Geometry: final body of the model. Coordinates: model frame, mm. Face numbers are marked on the shaded views. A direction names the side the tool comes from. Round coordinates to 2 decimals unless told otherwise and drop trailing zeros. Loops run counter-clockwise (first coordinate to the right, second up) from the corner with the lowest first, then second, coordinate; pieces in that order, holes last. Notation, with made-up numbers: (88.25, 30.5) -> (143.25, 30.5) arc R19 cw to (143.25, 55.5) -> close; hole circle Ø10 at (59, 17.25). An arc over 180 degrees is marked (long way). Answer in a Markdown table with one row per item.
Autodesk Inventor part; units mm, degrees
ref_plane "YZ Plane" through (0, 0, 0) normal (1, 0, 0) x (0, 1, 0)
ref_plane "XZ Plane" through (0, 0, 0) normal (0, 1, 0) x (-1, 0, 0)
ref_plane "XY Plane" through (0, 0, 0) normal (0, 0, 1) x (1, 0, 0)
sketch "Sketch11" plane through (0, 0, 0) normal (0, 1, 0) x (-1, 0, 0)
  circle A0 centre (0, 0) radius 26
  circle A1 centre (0, 0) radius 24
  circle A2 centre (0, 0) radius 31
  circle A3 centre (0, 0) radius 55
  line L0 (35.5726, 38.3198) -> (39.3254, 31.8198)
  line L1 (39.3254, 31.8198) -> (35.5726, 25.3198)
  line L2 (35.5726, 25.3198) -> (28.067, 25.3198)
  line L3 (28.067, 25.3198) -> (24.3143, 31.8198)
  line L4 (24.3143, 31.8198) -> (28.067, 38.3198)
  line L5 (28.067, 38.3198) -> (35.5726, 38.3198)
  line L6 (0, 0) -> (31.8198, 31.8198) construction
  line L7 (0, 0) -> (45, 0) construction
  line L8 (35.5726, 38.3198) -> (28.067, 25.3198) construction
  line L9 (28.067, 38.3198) -> (35.5726, 25.3198) construction
  line L10 (39.3254, 31.8198) -> (24.3143, 31.8198) construction
  line L11 (0, 52.6213) -> (0, 85)
  line L12 (0, 85) -> (-16, 85)
  line L13 (-16, 85) -> (-16, 52.6213)
  line L14 (0, 74.5) -> (120, 74.5)
  line L15 (120, 74.5) -> (120, 80)
  line L16 (120, 80) -> (0, 80)
  line L17 (0, 80) -> (0, 74.5)
  line L18 (120, 90.5) -> (120, 58.5)
  arc A4 (120, 58.5) -> (120, 90.5) centre (120, 74.5) ccw
  line L19 (-16, 52.6213) -> (0, 52.6213)
  line L20 (0, 52.6213) -> (-16, 52.6213)
  line L21 (-16, 52.6213) -> (-16, 44.6213)
  line L22 (-16, 44.6213) -> (0, 44.6213)
  line L23 (0, 44.6213) -> (0, 52.6213)
  dimension "oOuterDia" = 110
  dimension "oPipeDia" = 52
  dimension "oPipeWall" = 2
  dimension "oPipeLenght" = 5
  dimension "oKdia" = 45
  dimension "d70" = 45
  dimension "oSW" = 13
  dimension "oCenterTop" = 85
  dimension "d78" = 16
  dimension "oHandleLenght" = 120
  dimension "d80" = 5.5
  dimension "d81" = 32
  dimension "d82" = 5
  dimension "d86" = 8
extrude "Extrusion12" add sketch "Sketch11" along normal mid plane 52 contours A0
extrude "Extrusion13" add sketch "Sketch11" along normal mid plane 42 contours A2
extrude "Extrusion14" add sketch "Sketch11" along normal mid plane 22 contours L21 L22 L23 L11 A3 | A3 L11 L19 | L19 L23 L22 L21 | L0 L1 L2 L3 L4 L5
extrude "Extrusion15" add sketch "Sketch11" along normal mid plane 38 contours L0 L1 L2 L3 L4 L5
pattern_circular "Circular Pattern2" count 4 over 360 about axis through (0, 0, 0) along (0, 1, 0) of "Extrusion15"
revolve "Revolution1" add sketch "Sketch11" angle 360 about axis through (0, 0, 52.6213) along (0, 0, 1) contours L13 L12 L11 A3 | A3 L11 L19 | L19 L23 L22 L21
revolve "Revolution2" add sketch "Sketch11" angle 360 about axis through (0, 0, 74.5) along (-1, 0, 0) contours L11 L16 L15 L14
revolve "Revolution3" add sketch "Sketch11" angle 360 about axis through (-120, 0, 90.5) along (0, 0, -1) contours L15 L18 A4
equation "\"d65\" = -2 * oPipeLenght + oValveLenght"
properties part number "MANUAL SANITARY BUTTERFLY VALVE 304L DN50" material "304L"
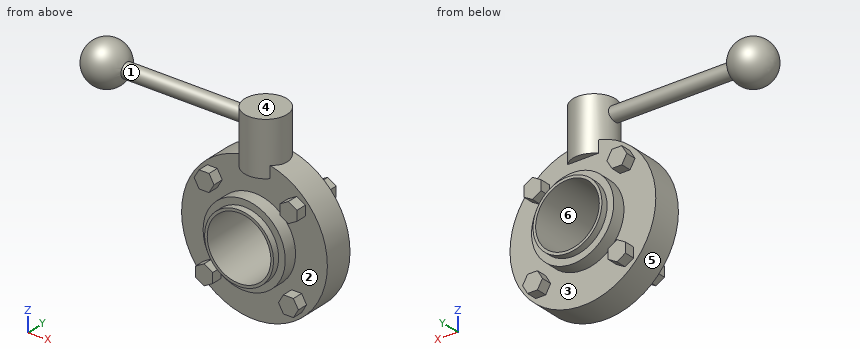
Item 1: Cut plane B-B (x = 0). Output: boundary loops of the cut face in (y, z).
Answer:
| item | result |
|---|---|
| outline | (-26, -26) -> (-21, -26) -> (-21, -31) -> (-11, -31) -> (-11, -55) -> (11, -55) -> (11, -31) -> (21, -31) -> (21, -26) -> (26, -26) -> (26, -24) -> (-26, -24) -> close; (-26, 24) -> (26, 24) -> (26, 26) -> (21, 26) -> (21, 31) -> (11, 31) -> (11, 44.62) -> (16, 44.62) -> (16, 85) -> (-16, 85) -> (-16, 44.62) -> (-11, 44.62) -> (-11, 31) -> (-21, 31) -> (-21, 26) -> (-26, 26) -> close |
Item 2: Pin query (flat end, axial travel): pin 1 Ø5 at (x, y) = (7.5, 14.5) entering from +Z; pin 2 Ø4 at (x, z) = (30.5, -30) entering from -Y; pin 3 Ø14.5 at (x, z) = (34.5, 29) entering from +Y. Return the tip coordinate at first contact, or that it passes through.
Answer:
| item | result |
|---|---|
| pin 1 | stops at z = 85 |
| pin 2 | stops at y = -19 |
| pin 3 | stops at y = 19 |
Item 3: Line query: probe 1 along Z at (x, y) = (0, 13.5); probe 2 along Y at (x, z) = (-23, 32); probe 3 along X at (y, z) = (-1, -11). Output: solid intervals per line, ascending. Write a range as [from, to].
Answer:
| item | result |
|---|---|
| probe 1 | z = [-31, -24], [24, 31], [44.62, 85] |
| probe 2 | y = [-11, 11] |
| probe 3 | x = [-53.89, -21.33], [21.33, 53.89] |
Item 4: Reachability of the marked faces 1, 2 and 3 from +Z, -Z, +X, -X, +Y, -Y: full face, straight path, thin tool, end or side. Return the list, or none.
Answer:
| item | result |
|---|---|
| face 1 | none |
| face 2 | -Y |
| face 3 | +Y |
Item 5: Draft query along Z for the marked faces 4, 5 and 6. Return one class per face: pulls with the +Z half, pulls with the -Z half, needs draft (parallel to the pull), parting line crosses it, or undercut.
Answer:
| item | result |
|---|---|
| face 4 | pulls with the +Z half |
| face 5 | undercut |
| face 6 | undercut |
Item 6: Cut plane D-D (x = -70). Output: boundary loops of the cut face in (y, z), then the cut area to 3 significant figures.
Answer:
| item | result |
|---|---|
| outline | circle Ø11 at (0, 74.5) |
| area | 95.0 mm² |
Item 7: Cut plane A-A (z = 0). Output: boundary loops of the cut face in (x, y), then the cut area to 3 significant figures.
Answer:
| item | result |
|---|---|
| outline | (-55, -11) -> (-31, -11) -> (-31, -21) -> (-26, -21) -> (-26, -26) -> (-24, -26) -> (-24, 26) -> (-26, 26) -> (-26, 21) -> (-31, 21) -> (-31, 11) -> (-55, 11) -> close; (24, -26) -> (26, -26) -> (26, -21) -> (31, -21) -> (31, -11) -> (55, -11) -> (55, 11) -> (31, 11) -> (31, 21) -> (26, 21) -> (26, 26) -> (24, 26) -> close |
| area | 1,680 mm² |
Item 8: Cut plane C-C (y = -2). Output: boundary loops of the cut face in (x, z), then the cut area to 3 significant figures.
Answer:
| item | result |
|---|---|
| outline | (-104.98, 69.38) -> (-15.87, 69.38) -> (-15.87, 52.66) arc R55 ccw (long way) to (15.87, 52.66) -> (15.87, 85) -> (-15.87, 85) -> (-15.87, 79.62) -> (-104.98, 79.62) arc R15.87 ccw (long way) to start; hole circle Ø48 at (0, 0) |
| area | 10,400 mm² |
